from build123d import *

# Parameters (mm, degrees)
BOX108_W        = 3
BOX108_H        = 6
BOX108_DEPTH    = 10
FILLET029_R     = 1.49
BOX107_W        = 3
BOX107_H        = 6
BOX107_DEPTH    = 10
FILLET028_R     = 1.49
BOX106_W        = 18
BOX106_H        = 81
BOX106_DEPTH    = 2
BOX105_W        = 18
BOX105_H        = 10
BOX105_DEPTH    = 10
BOX104_W        = 18
BOX104_H        = 10
BOX104_DEPTH    = 10
CHAMFER014_SIZE = 1.99


with BuildPart() as fillet029:
    # Box108 → Box108 (new body)
    with BuildSketch(Plane.XY):
        with Locations((1.5, 3)):
            Rectangle(BOX108_W, BOX108_H)
    extrude(amount=BOX108_DEPTH)

    # Fillet029
    fillet029_edges = [fillet029.edges().sort_by_distance(p)[0] for p in [
        (0, 0, 5),
        (0, 6, 5),
        (3, 0, 5),
        (3, 6, 5),
    ]]
    fillet(fillet029_edges, radius=FILLET029_R)


with BuildPart() as fillet029_1:
    # Fillet029 placement: moved
    add(fillet029.part.moved(Location((31, 59.5, -6))))


with BuildPart() as fusion133:
    # Box107 → Box107 (new body)
    with BuildSketch(Plane.XY):
        with Locations((1.5, 3)):
            Rectangle(BOX107_W, BOX107_H)
    extrude(amount=BOX107_DEPTH)

    # Fillet028
    fillet028_edges = [fusion133.edges().sort_by_distance(p)[0] for p in [
        (0, 0, 5),
        (0, 6, 5),
        (3, 0, 5),
        (3, 6, 5),
    ]]
    fillet(fillet028_edges, radius=FILLET028_R)


with BuildPart() as fusion133_1:
    # Fillet028 placement: moved
    add(fusion133.part.moved(Location((31, 15.5, -6))))

    # Fusion133: union Fillet029
    add(fillet029_1.part)


with BuildPart() as cube078:
    # Box106 → Box106 (new body)
    with BuildSketch(Plane(origin=(27, 0, -2), x_dir=(1, 0, 0), z_dir=(0, 0, 1))):
        with Locations((9, 40.5)):
            Rectangle(BOX106_W, BOX106_H)
    extrude(amount=BOX106_DEPTH)


with BuildPart() as cube077:
    # Box105 → Box105 (new body)
    with BuildSketch(Plane(origin=(27, 71, -10), x_dir=(1, 0, 0), z_dir=(0, 0, 1))):
        with Locations((9, 5)):
            Rectangle(BOX105_W, BOX105_H)
    extrude(amount=BOX105_DEPTH)


with BuildPart() as kipper_frame_missing_part:
    # Box104 → Box104 (new body)
    with BuildSketch(Plane(origin=(27, 0, -10), x_dir=(1, 0, 0), z_dir=(0, 0, 1))):
        with Locations((9, 5)):
            Rectangle(BOX104_W, BOX104_H)
    extrude(amount=BOX104_DEPTH)

    # Fusion132: union Cube078, Cube077
    add(cube078.part)
    add(cube077.part)

    # Cut125: cut Fusion133
    add(fusion133_1.part, mode=Mode.SUBTRACT)

    # Chamfer014
    chamfer014_edges = [kipper_frame_missing_part.edges().sort_by_distance(p)[0] for p in [
        (27, 40.5, -2),
        (45, 40.5, -2),
    ]]
    chamfer(chamfer014_edges, length=CHAMFER014_SIZE)


with BuildPart() as kipper_frame_missing_part_1:
    # Chamfer014 placement: moved
    add(kipper_frame_missing_part.part.moved(Location((0, -0.5, 0))))


solid = kipper_frame_missing_part_1.part
The model under review builds one solid part; all positions refer to its coordinate system, in mm. A direction names the side the tool comes from. Give positions to 0.01 mm unless a question says otherwise; leave off trailing zeros. Loops run counter-clockwise (first coordinate to the right, second up) from the corner with the lowest first, then second, coordinate; pieces in that order, holes last. Notation, with made-up numbers: (68.5, -24.75) -> (112.5, -24.75) arc R11 ccw to (112.5, -15.75) -> close; hole circle Ø1 at (74.5, 34). An arc over 180 degrees is marked (long way). Put each result on its own line as item: value. Start each with the question number.
1. Clearance check with flat-ended pins moving along their axes: P1, Ø0.6, axis at y = 61.5, z = -0.5, coming from the +X side; P2, Ø1.6, axis at y = 18.5, z = -1, coming from the -X side; P3, Ø1, axis at y = 17.5, z = -1, coming from the +X side. State where each tip first meets the part, or that it passes through.
2. Wall thickness on probe 1 along Y at (x, z) = (34, -4.5); probe 2 along Z at (x, y) = (36.25, 38.5); probe 3 along Z at (x, y) = (44, 62): over which ranges is each line inside the solid? List them lowest first.
3. We need section B-B on z = -0.75. State how many separate pieces and enclosed holes the cut face has, then the cut area to 3 significant figures.
4. For faces 1 (the face through (36, 5, -10)), 2 (the face through (33.575, 20.552, -0.986)), 3 (the face through (36, 40, -2)), list the 3-axis set-ups (+Z, -Z, +X, -X, +Y, -Y) from which the entire face can be reached by the end or side of a thin tool; tool diameter is ignored.
5. We need section A-A on z = -9. State the section outline as (x, y) points, then the cut area to 3 significant figures.
6. We need section C-C on x = 37.5. State the section outline as (y, z) points.
7. Mouldability with a two-part tool opening along X and no side actions: class faces 4 (the face through (31.425, 59.448, -0.986)), 5 (the face through (44.02, 39.57, -0.99)), 6 (the face through (36, 41, 0)), 7 (the face through (28.01, 39.57, -1.02)) as released by +X, released by -X, zero draft, split by the parting line, or undercut.
Determined:
1. P1: x = 44.81
1. P2: x = 27.19
1. P3: x = 44.51
2. probe 1: -0.5 to 9.5, 70.5 to 80.5
2. probe 2: -2 to 0
2. probe 3: -1.01 to 0
3. separate pieces: 1
3. enclosed holes: 2
3. area: 1,340 mm^2
4. face 1: -Z, +X, -X, +Y, -Y
4. face 2: +Z, -Z
4. face 3: -Z, +X, -X
5. outline: (27, -0.5) -> (45, -0.5) -> (45, 9.5) -> (27, 9.5) -> close; (27, 70.5) -> (45, 70.5) -> (45, 80.5) -> (27, 80.5) -> close
5. area: 360 mm^2
6. outline: (-0.5, -10) -> (9.5, -10) -> (9.5, -2) -> (70.5, -2) -> (70.5, -10) -> (80.5, -10) -> (80.5, 0) -> (-0.5, 0) -> close
7. face 4: undercut
7. face 5: released by +X
7. face 6: zero draft
7. face 7: released by -X
